```python
from build123d import *

# Parameters (mm, degrees)
SKETCH1_R               = 7.5
BOSS_EXTRUDE1_DEPTH     = 24
CUT_EXTRUDE1_DEPTH      = 27.239283527
CUT_EXTRUDE1_DEPTH_BACK = 27.239283527
SKETCH2_R               = 5.1


with BuildPart() as part:
    # Sketch1 → Boss-Extrude1 (new body)
    with BuildSketch(Plane(origin=(0, 0, 0), x_dir=(1, 0, 0), z_dir=(0, 1, 0))):
        with Locations(Location((0, 0, 0), (0, 0, 270))):
            Circle(SKETCH1_R)
    extrude(amount=BOSS_EXTRUDE1_DEPTH)

    # Sketch2 → Cut-Extrude1 (cut, two sides: drawn at the far end of the back side and taken through both)
    with BuildSketch(Plane.XY.offset(-CUT_EXTRUDE1_DEPTH_BACK)):
        with Locations(Location((0, 12, 0), (0, 0, 90.000000001))):
            Circle(SKETCH2_R)
    extrude(amount=CUT_EXTRUDE1_DEPTH + CUT_EXTRUDE1_DEPTH_BACK, mode=Mode.SUBTRACT)

    # Sketch3 → Revolve1 (revolve)
    with BuildSketch(Plane.XY, mode=Mode.PRIVATE) as revolve1_sk:
        Polygon((0, 24), (-7.5, 24), (-7.5, 25), (-6.5, 25), (-6.5, 26.1), (-7.5, 26.1), (-7.5, 27), (0, 27), align=None)
        Polygon((-7.5, -3), (0, -3), (0, 0), (-7.5, 0), (-7.5, -1), (-6.5, -1), (-6.5, -2.1), (-7.5, -2.1), align=None)
    revolve(revolve1_sk.sketch.rotate(Axis((0, 0, 0), (0, 1, 0)), 270), axis=Axis((0, 0, 0), (0, 1, 0)))


solid = part.part
```
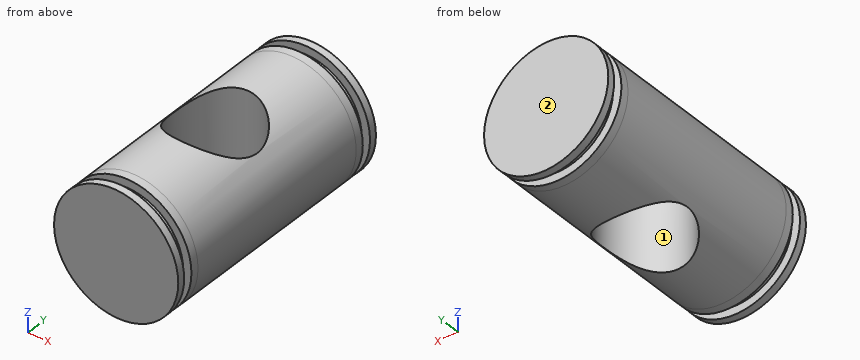
Here's how the part is built. I have some questions about the finished solid (model axes, mm). Face numbers are marked on the shaded views. Give positions to 0.01 mm unless a question says otherwise; leave off trailing zeros. Loops run counter-clockwise (first coordinate to the right, second up) from the corner with the lowest first, then second, coordinate; pieces in that order, holes last. Notation, with made-up numbers: M 53.25,64 L 99.25,64 A33 cw 99.25,97 Z; hole C 29.5,29 d6. An arc over 180 degrees is marked long. Put each result on its own line as item: value. Start each with the question number.
(1) I want a section at D-D on x = -6. Please give me the cut outline in (y, z), then the cut area to 3 significant figures.
(2) I want a section at A-A on x = 0. Please give me the cut outline in (y, z).
(3) If we mould it in two halves opening along X, with no side actions, what happens to the marked faces 1 and 2? For each: +X half, -X half, draft (parallel to the pull), parting line (faces both ways), or undercut.
(4) Will these pins go through, and if not, where does the flat tip stop? pin 1 Ø3 at (x, y) = (3, 3) entering from +Z; pin 2 Ø1.5 at (x, y) = (1, 18.5) entering from -Z; pin 3 Ø1.5 at (x, y) = (-5.5, 10.5) entering from -Z; pin 4 Ø4 at (x, y) = (1.5, 22.5) entering from +Z.
(5) I want a section at B-B on z = 0. Please give me the cut outline in (x, y).
(6) I need wall thicknesses on line 1 along Y through (x, z) = (0, 4.75); line 2 along X through (y, z) = (12, -3.75); line 3 along Y through (x, z) = (-2.5, 0.75). Which ranges of each line are inside material? Lowest first, please. Write a range as [from, to].
Answer block:
1. outline: M -3,-4.5 L -2.1,-4.5 L -2.1,-2.5 L -1,-2.5 L -1,-4.5 L 25,-4.5 L 25,-2.5 L 26.1,-2.5 L 26.1,-4.5 L 27,-4.5 L 27,4.5 L 26.1,4.5 L 26.1,2.5 L 25,2.5 L 25,4.5 L -1,4.5 L -1,2.5 L -2.1,2.5 L -2.1,4.5 L -3,4.5 Z
1. area: 261 mm^2
2. outline: M -3,-7.5 L -2.1,-7.5 L -2.1,-6.5 L -1,-6.5 L -1,-7.5 L 6.9,-7.5 L 6.9,7.5 L -1,7.5 L -1,6.5 L -2.1,6.5 L -2.1,7.5 L -3,7.5 Z; M 17.1,-7.5 L 25,-7.5 L 25,-6.5 L 26.1,-6.5 L 26.1,-7.5 L 27,-7.5 L 27,7.5 L 26.1,7.5 L 26.1,6.5 L 25,6.5 L 25,7.5 L 17.1,7.5 Z
3. face 1: undercut
3. face 2: draft
4. pin 1: z = 7.35
4. pin 2: z = -7.5
4. pin 3: z = -5.77
4. pin 4: z = 7.5
5. outline: M -7.5,-3 L 7.5,-3 L 7.5,-2.1 L 6.5,-2.1 L 6.5,-1 L 7.5,-1 L 7.5,25 L 6.5,25 L 6.5,26.1 L 7.5,26.1 L 7.5,27 L -7.5,27 L -7.5,26.1 L -6.5,26.1 L -6.5,25 L -7.5,25 L -7.5,-1 L -6.5,-1 L -6.5,-2.1 L -7.5,-2.1 Z; hole C 0,12 d10.2
6. line 1: [-3, 6.9], [17.1, 27]
6. line 2: [-6.5, -5.1], [5.1, 6.5]
6. line 3: [-3, 7.55], [16.45, 27]
